```python
from build123d import *

# Parameters (mm, degrees)
SKETCH1_W           = 228.6
SKETCH1_H           = 177.8
BOSS_EXTRUDE1_DEPTH = 3.175
SKETCH2_R           = 2.1717
SKETCH2_R_2         = 3.175
SKETCH2_R_3         = 22.352
SKETCH2_R_4         = 2.159
SKETCH2_W           = 60.96
SKETCH2_H           = 25.4
CUT_EXTRUDE1_DEPTH  = 3.175


with BuildPart() as part:
    # Sketch1 → Boss-Extrude1 (new body)
    with BuildSketch(Plane(origin=(0, 0, 0), x_dir=(1, 0, 0), z_dir=(0, 1, 0))):
        with Locations((-103.587357149, -18.25946167)):
            Rectangle(SKETCH1_W, SKETCH1_H)
    extrude(amount=BOSS_EXTRUDE1_DEPTH)

    # Sketch2 → Cut-Extrude1 (cut)
    with BuildSketch(Plane(origin=(0, 3.175, 0), x_dir=(1, 0, 0), z_dir=(0, 1, 0))):
        with Locations(Location((4.362642851, 35.08053833, 0), (0, 0, 270))):
            Circle(SKETCH2_R)
        with Locations(Location((-25.355357149, 35.08053833, 0), (0, 0, 270))):
            Circle(SKETCH2_R)
        with Locations(Location((4.362642851, -71.59946167, 0), (0, 0, 270))):
            Circle(SKETCH2_R)
        with Locations(Location((-25.355357149, -71.59946167, 0), (0, 0, 270))):
            Circle(SKETCH2_R)
        with Locations(Location((-207.727357149, 42.70053833, 0), (0, 0, 270))):
            Circle(SKETCH2_R_2)
        with Locations(Location((-152.660157149, 42.70053833, 0), (0, 0, 270))):
            Circle(SKETCH2_R_2)
        with Locations(Location((-180.193757149, 42.70053833, 0), (0, 0, 270))):
            Circle(SKETCH2_R_3)
        with Locations(Location((-207.727357149, -79.21946167, 0), (0, 0, 270))):
            Circle(SKETCH2_R_2)
        with Locations(Location((-180.193757149, -79.21946167, 0), (0, 0, 270))):
            Circle(SKETCH2_R_3)
        with Locations(Location((-152.660157149, -79.21946167, 0), (0, 0, 270))):
            Circle(SKETCH2_R_2)
        with Locations(Location((-54.692357149, 49.24054303, 0), (0, 0, 270))):
            Circle(SKETCH2_R)
        with Locations(Location((-125.558357149, 49.24054303, 0), (0, 0, 270))):
            Circle(SKETCH2_R)
        with Locations(Location((-125.558357149, -85.75946637, 0), (0, 0, 270))):
            Circle(SKETCH2_R)
        with Locations(Location((-54.692357149, -85.75946637, 0), (0, 0, 270))):
            Circle(SKETCH2_R)
        with Locations(Location((-54.057357149, 66.83053833, 0), (0, 0, 270))):
            Circle(SKETCH2_R_4)
        with Locations(Location((-54.057357149, -103.34946167, 0), (0, 0, 270))):
            Circle(SKETCH2_R_4)
        with Locations(Location((-214.077357149, 66.83053833, 0), (0, 0, 270))):
            Circle(SKETCH2_R_4)
        with Locations(Location((-214.077357149, -103.34946167, 0), (0, 0, 270))):
            Circle(SKETCH2_R)
        with Locations(Location((-79.457357149, 66.83053833, 0), (0, 0, 270))):
            Circle(SKETCH2_R)
        with Locations(Location((-104.857357149, 66.83053833, 0), (0, 0, 270))):
            Circle(SKETCH2_R)
        with Locations(Location((-130.257357149, 66.83053833, 0), (0, 0, 270))):
            Circle(SKETCH2_R)
        with Locations(Location((-155.657357149, 66.83053833, 0), (0, 0, 270))):
            Circle(SKETCH2_R)
        with Locations(Location((-79.457357149, -103.34946167, 0), (0, 0, 270))):
            Circle(SKETCH2_R)
        with Locations(Location((-104.857357149, -103.34946167, 0), (0, 0, 270))):
            Circle(SKETCH2_R)
        with Locations(Location((-130.257357149, -103.34946167, 0), (0, 0, 270))):
            Circle(SKETCH2_R)
        with Locations(Location((-155.657357149, -103.34946167, 0), (0, 0, 270))):
            Circle(SKETCH2_R)
        with Locations(Location((-214.077357149, 19.84053833, 0), (0, 0, 270))):
            Circle(SKETCH2_R)
        with Locations(Location((-214.077357149, -5.55946167, 0), (0, 0, 270))):
            Circle(SKETCH2_R)
        with Locations(Location((-214.077357149, -30.95946167, 0), (0, 0, 270))):
            Circle(SKETCH2_R)
        with Locations(Location((-214.077357149, -56.35946167, 0), (0, 0, 270))):
            Circle(SKETCH2_R)
        with Locations(Location((-130.257357149, 19.84053833, 0), (0, 0, 270))):
            Circle(SKETCH2_R)
        with Locations(Location((-130.257357149, -56.35946167, 0), (0, 0, 270))):
            Circle(SKETCH2_R)
        with Locations(Location((6.902642851, 19.84053833, 0), (0, 0, 270))):
            Circle(SKETCH2_R)
        with Locations(Location((6.902642851, -5.55946167, 0), (0, 0, 270))):
            Circle(SKETCH2_R)
        with Locations(Location((6.902642851, -30.95946167, 0), (0, 0, 270))):
            Circle(SKETCH2_R)
        with Locations(Location((6.902642851, -56.35946167, 0), (0, 0, 270))):
            Circle(SKETCH2_R)
        with Locations(Location((-54.057357149, 19.84053833, 0), (0, 0, 270))):
            Circle(SKETCH2_R)
        with Locations(Location((-54.057357149, -56.35946167, 0), (0, 0, 270))):
            Circle(SKETCH2_R)
        with Locations((-19.767357149, -94.45946167)):
            Rectangle(SKETCH2_W, SKETCH2_H)
        with Locations((-19.767357149, 57.94053833)):
            Rectangle(SKETCH2_W, SKETCH2_H)
    extrude(amount=-CUT_EXTRUDE1_DEPTH, mode=Mode.SUBTRACT)


solid = part.part
```
Work out the finished part from the listing and answer in its coordinate system (mm). Give positions to 0.01 mm unless a question says otherwise; leave off trailing zeros. Order: outer loops, then holes, each group sorted by start corner. A loop starts at its lowest first (then second) coordinate and runs counter-clockwise, first axis right, second up. Notation, with made-up numbers: M -17,-15 L -6,-15 A26 cw -6,1 Z; hole C 16.25,-10.75 d8. An arc over 180 degrees is marked long. Return JSON: item names as keys, results as strings.
1) Each of these flat-tipped pins is pushed along its axis until it touches: pin 1 (2.5 mm diameter, centred on x = -25.36, z = 71.6, fed in from +Y); pin 2 (1 mm diameter, centred on x = -43, y = 2, fed in from +Z). Where does it stop, or does it pass through?
Resolved:
{"pin 1": "through", "pin 2": "z = 81.76"}
2) For a pull along Z with two mould halves and no side action, classify faces 1 (the flat face through (-105, 3.175, 17)), 2 (the cylindrical face through (-200.024, 1.61, -32.386)) as +Z half, -Z half, draft (parallel to the pull), parting line (faces both ways), or undercut.
Resolved:
{"face 1": "draft", "face 2": "undercut"}
3) Section C-C, the plane x = -34 is taken. Write down the section's boundary in (y, z) (3 decimals).
Resolved:
{"outline": "M 0,-45.241 L 3.175,-45.241 L 3.175,81.759 L 0,81.759 Z"}
4) Section B-B, the plane y = 2.15 is taken. Give the number of separate pieces and of enclosed holes in the cut face, plus the area to 3 significant figures.
Resolved:
{"separate pieces": "1", "enclosed holes": "38", "area": "33,800 mm^2"}
5) Section A-A, the plane x = -199 is taken. Write down the section's boundary in (y, z) (3 decimals), plus the area to 3 significant figures.
Resolved:
{"outline": "M 0,-70.641 L 3.175,-70.641 L 3.175,-54.781 L 0,-54.781 Z; M 0,-30.62 L 3.175,-30.62 L 3.175,67.139 L 0,67.139 Z; M 0,91.3 L 3.175,91.3 L 3.175,107.159 L 0,107.159 Z", "area": "411 mm^2"}
6) Straight lines are drawn through the part: line 1 along X through (y, z) = (0.65, 31); line 2 along X through (y, z) = (0.2, 87); line 3 along Z through (x, y) = (-161, 1.7). For each, find the intervals that lie inside material, in ascending order. Write a range as [from, to].
Resolved:
{"line 1": "[-217.89, -216.25], [-211.91, 4.73], [9.07, 10.71]", "line 2": "[-217.89, -201.15], [-159.24, -127.34], [-123.78, -56.47], [-52.91, -50.25]", "line 3": "[-70.64, -54.16], [-31.25, 67.76], [90.67, 107.16]"}
